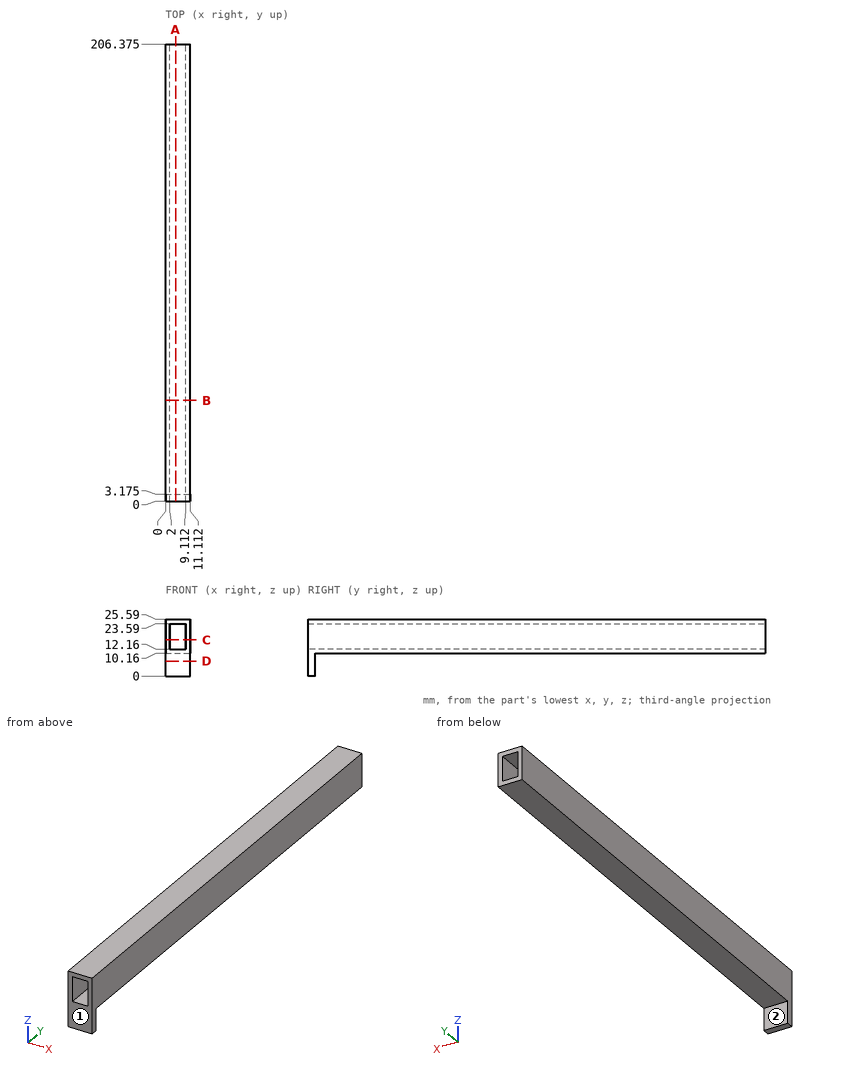
Job drawing, mm, ordinate dimensions from the low corner. One solid piece. A direction names the side the tool comes from. Round coordinates to 2 decimals unless told otherwise and drop trailing zeros. Write each loop counter-clockwise with the first axis right and the second up, starting at its lowest first coordinate (ties: lowest second). Pieces come first, ordered by that corner, then holes.
1) Band-saw the part on C-C, the plane z = 16.25. List the corners of the cut face in (x, y) (3 decimals), and give its area (4 significant figures).
2) Pin check, flat tips, straight feed: pin 1 (2 mm diameter, centred on x = 2.5, z = 2.5, fed in from +Y) (3 decimals); pin 2 (3.5 mm diameter, centred on x = 3.5, y = 113.5, fed in from -Z). Stop position of each tip, or through.
3) Drill centre lines: probe 1 along Z at (x, y) = (4, 130.5); probe 2 along X at (y, z) = (62, 23.5); probe 3 along Z at (x, y) = (9.75, 196.5). Where is each one in solid material? Low to high.
4) Band-saw the part on A-A, the plane x = 4.5. List the corners of the cut face in (y, z) (3 decimals), and give its area (3 significant figures).
5) 3-axis set-ups, long thin cutter, end or side, ignore diameter. For the marked faces 1 and 2: which of +Z, -Z, +X, -X, +Y, -Y reach the whole face in a straight line?
6) Band-saw the part on D-D, the plane z = 6.75. List the corners of the cut face in (x, y) (3 decimals), and give its area (3 significant figures).
7) Band-saw the part on B-B, the plane y = 45.5. List the corners of the cut face in (x, z), and give its area (3 significant figures).
Ans:
1. outline: (0, 0) - (2, 0) - (2, 206.375) - (0, 206.375) - close; (9.112, 0) - (11.112, 0) - (11.112, 206.375) - (9.112, 206.375) - close
1. area: 825.5 mm2
2. pin 1: stops at y = 3.175
2. pin 2: stops at z = 10.16
3. probe 1: z = 10.16 to 12.16, 23.59 to 25.59
3. probe 2: x = 0 to 2, 9.11 to 11.11
3. probe 3: z = 10.16 to 25.59
4. outline: (0, 0) - (3.175, 0) - (3.175, 10.16) - (206.375, 10.16) - (206.375, 12.16) - (0, 12.16) - close; (0, 23.59) - (206.375, 23.59) - (206.375, 25.59) - (0, 25.59) - close
4. area: 858 mm2
5. face 1: +Z, -Z, +X, -X, -Y
5. face 2: -Z, +X, -X, +Y
6. outline: (0, 0) - (11.112, 0) - (11.112, 3.175) - (0, 3.175) - close
6. area: 35.3 mm2
7. outline: (0, 10.16) - (11.11, 10.16) - (11.11, 25.59) - (0, 25.59) - close; hole (2, 12.16) - (9.11, 12.16) - (9.11, 23.59) - (2, 23.59) - close
7. area: 90.2 mm2
